```python
from build123d import *

# Parameters (mm, degrees)
BOSS_EXTRUDE3_DEPTH = 120
FILLET4_R           = 1


with BuildPart() as part:
    # Sketch5 → Boss-Extrude3 (new body)
    with BuildSketch(Plane.XY):
        with BuildLine():
            Line((-2.689552127, 0.955752212), (88.310447873, 0.955752212))
            ThreePointArc((88.310447873, 0.955752212), (90.078214826, 1.687985259), (90.810447873, 3.455752212))
            Line((90.810447873, 3.455752212), (90.810447873, 18.955752212))
            Line((90.810447873, 18.955752212), (92.810447873, 18.955752212))
            Line((92.810447873, 18.955752212), (92.810447873, 2.955752212))
            Line((92.810447873, 2.955752212), (92.810447873, 1.455752212))
            ThreePointArc((92.810447873, 1.455752212), (92.078214826, -0.312014741), (90.310447873, -1.044247788))
            Line((90.310447873, -1.044247788), (-4.689552127, -1.044247788))
            ThreePointArc((-4.689552127, -1.044247788), (-6.45731908, -0.312014741), (-7.189552127, 1.455752212))
            Line((-7.189552127, 1.455752212), (-7.189552127, 2.955752212))
            Line((-7.189552127, 2.955752212), (-7.189552127, 18.955752212))
            Line((-7.189552127, 18.955752212), (-5.189552127, 18.955752212))
            Line((-5.189552127, 18.955752212), (-5.189552127, 3.455752212))
            ThreePointArc((-5.189552127, 3.455752212), (-4.45731908, 1.687985259), (-2.689552127, 0.955752212))
        make_face()
    extrude(amount=BOSS_EXTRUDE3_DEPTH)

    # Fillet4
    fillet4_edges = [part.edges().sort_by_distance(p)[0] for p in [
        (92.810447873, 18.955752212, 60),
        (90.810447873, 18.955752212, 60),
        (-7.189552127, 18.955752212, 60),
        (-5.189552127, 18.955752212, 60),
    ]]
    fillet(fillet4_edges, radius=FILLET4_R - 0.0001)  # a hair under: the kernel refuses the full size


solid = part.part
```
Verification items for the finished model (mm, model axes). A direction names the side the tool comes from. Coordinates: 2 decimals unless noted, no trailing zeros. Loops run counter-clockwise (first coordinate to the right, second up) from the corner with the lowest first, then second, coordinate; pieces in that order, holes last. Notation, with made-up numbers: (14.5, 65.25) -> (68.5, 65.25) arc R20 ccw to (68.5, 78.25) -> close; hole circle Ø4 at (51, -19). An arc over 180 degrees is marked (long way). Answer in a Markdown table with one row per item. Add a question column.
1. Access from +Z, -Z, +X, -X, +Y, -Y to the whole of each face (thin tool, end or side, straight path). Record for faces 1 (the face through (92.1, -0.29, 59.16)), 2 (the face through (42, 0.956, 59)).
2. Depth check by flat-ended pin: P1, Ø2, axis at y = 1, z = 70.5, coming from the -X side. Enter the tip coordinate at first touch or a pass-through.
3. Material ranges on probe 1 along X at (y, z) = (11, 60); probe 2 along Y at (x, z) = (50, 101.5); probe 3 along X at (y, z) = (2.75, 98), recorded low to high. Write a range as [from, to].
4. Draft check along X on faces 3 (the face through (43, -1.044, 59)), 4 (the face through (90.81, 11, 59)), 5 (the face through (92.81, 10, 59)), 6 (the face through (-7.19, 10, 59)). Enter one of: +X half, -X half, draft (parallel to the pull), parting line (faces both ways), or undercut.
5. Section check A-A, the plane y = 11. Enter the section's corners in (x, z).
6. Section check C-C, the plane x = 21.5. Enter the section's corners in (y, z).
Derived:
| question | item | result |
|---|---|---|
| 1 | face 1 | +Z, -Z, +X, -Y |
| 1 | face 2 | +Z, -Z, +Y |
| 2 | P1 | stops at x = -7.19 |
| 3 | probe 1 | x = [-7.19, -5.19], [90.81, 92.81] |
| 3 | probe 2 | y = [-1.04, 0.96] |
| 3 | probe 3 | x = [-7.19, -5.09], [90.71, 92.81] |
| 4 | face 3 | draft |
| 4 | face 4 | undercut |
| 4 | face 5 | +X half |
| 4 | face 6 | -X half |
| 5 | outline | (-7.19, 0) -> (-5.19, 0) -> (-5.19, 120) -> (-7.19, 120) -> close; (90.81, 0) -> (92.81, 0) -> (92.81, 120) -> (90.81, 120) -> close |
| 6 | outline | (-1.04, 0) -> (0.96, 0) -> (0.96, 120) -> (-1.04, 120) -> close |
